Design review of the part built by this model. Coordinates are the model's own, in mm. Face numbers are marked on the shaded views. A direction names the side the tool comes from. Give positions to 0.01 mm unless a question says otherwise; leave off trailing zeros. Loops run counter-clockwise (first coordinate to the right, second up) from the corner with the lowest first, then second, coordinate; pieces in that order, holes last. Notation, with made-up numbers: (87, 21) - (143, 21) arc R24 ccw to (143, 39) - close; hole circle Ø7 at (55, 60.5). An arc over 180 degrees is marked (long way). Write each question's results on one line, items separated by ' | '.
```python
from build123d import *

# Parameters (mm, degrees)
SKETCH2_R           = 40
BOSS_EXTRUDE1_DEPTH = 20
SKETCH3_W           = 5.5
SKETCH3_H           = 4.31
SKETCH3_W_2         = 4.31
SKETCH3_H_2         = 5.5
CUT_EXTRUDE1_DEPTH  = 20
SKETCH4_R           = 6
CUT_EXTRUDE2_DEPTH  = 20


with BuildPart() as part:
    # Sketch2 → Boss-Extrude1 (new body)
    with BuildSketch(Plane.XY):
        Circle(SKETCH2_R)
    extrude(amount=BOSS_EXTRUDE1_DEPTH)

    # Sketch3 → Cut-Extrude1 (cut)
    with BuildSketch(Plane.XY):
        Polygon((-6.648248649, -35.436785829), (-7.763758734, -39.59992614), (-13.076350778, -38.176421392), (-11.960840694, -34.013281081), align=None)
        with Locations((0, -38.105)):
            Rectangle(SKETCH3_W, SKETCH3_H)
        Polygon((-15.59343014, -32.508613266), (-17.74843014, -36.241182756), (-22.51156986, -33.491182756), (-20.35656986, -29.758613266), align=None)
        Polygon((-23.475945135, -27.365032432), (-26.523575362, -30.412662659), (-30.412662659, -26.523575362), (-27.365032432, -23.475945135), align=None)
        Polygon((-29.758613266, -20.35656986), (-33.491182756, -22.51156986), (-36.241182756, -17.74843014), (-32.508613266, -15.59343014), align=None)
        Polygon((-34.013281081, -11.960840694), (-38.176421392, -13.076350778), (-39.59992614, -7.763758734), (-35.436785829, -6.648248649), align=None)
        with Locations((-38.105, 0)):
            Rectangle(SKETCH3_W_2, SKETCH3_H_2)
        Polygon((-35.436785829, 6.648248649), (-39.59992614, 7.763758734), (-38.176421392, 13.076350778), (-34.013281081, 11.960840694), align=None)
        Polygon((-32.508613266, 15.59343014), (-36.241182756, 17.74843014), (-33.491182756, 22.51156986), (-29.758613266, 20.35656986), align=None)
        Polygon((-27.365032432, 23.475945135), (-30.412662659, 26.523575362), (-26.523575362, 30.412662659), (-23.475945135, 27.365032432), align=None)
        Polygon((-20.35656986, 29.758613266), (-22.51156986, 33.491182756), (-17.74843014, 36.241182756), (-15.59343014, 32.508613266), align=None)
        Polygon((-11.960840694, 34.013281081), (-13.076350778, 38.176421392), (-7.763758734, 39.59992614), (-6.648248649, 35.436785829), align=None)
        with Locations((0, 38.105)):
            Rectangle(SKETCH3_W, SKETCH3_H)
        Polygon((6.648248649, 35.436785829), (7.763758734, 39.59992614), (13.076350778, 38.176421392), (11.960840694, 34.013281081), align=None)
        Polygon((15.59343014, 32.508613266), (17.74843014, 36.241182756), (22.51156986, 33.491182756), (20.35656986, 29.758613266), align=None)
        Polygon((23.475945135, 27.365032432), (26.523575362, 30.412662659), (30.412662659, 26.523575362), (27.365032432, 23.475945135), align=None)
        Polygon((29.758613266, 20.35656986), (33.491182756, 22.51156986), (36.241182756, 17.74843014), (32.508613266, 15.59343014), align=None)
        Polygon((34.013281081, 11.960840694), (38.176421392, 13.076350778), (39.59992614, 7.763758734), (35.436785829, 6.648248649), align=None)
        with Locations((38.105, 0)):
            Rectangle(SKETCH3_W_2, SKETCH3_H_2)
        Polygon((35.436785829, -6.648248649), (39.59992614, -7.763758734), (38.176421392, -13.076350778), (34.013281081, -11.960840694), align=None)
        Polygon((32.508613266, -15.59343014), (36.241182756, -17.74843014), (33.491182756, -22.51156986), (29.758613266, -20.35656986), align=None)
        Polygon((27.365032432, -23.475945135), (30.412662659, -26.523575362), (26.523575362, -30.412662659), (23.475945135, -27.365032432), align=None)
        Polygon((20.35656986, -29.758613266), (22.51156986, -33.491182756), (17.74843014, -36.241182756), (15.59343014, -32.508613266), align=None)
        Polygon((11.960840694, -34.013281081), (13.076350778, -38.176421392), (7.763758734, -39.59992614), (6.648248649, -35.436785829), align=None)
    extrude(amount=CUT_EXTRUDE1_DEPTH, mode=Mode.SUBTRACT)

    # Sketch4 → Cut-Extrude2 (cut)
    with BuildSketch(Plane.XY):
        Circle(SKETCH4_R)
    extrude(amount=CUT_EXTRUDE2_DEPTH, mode=Mode.SUBTRACT)


solid = part.part
```
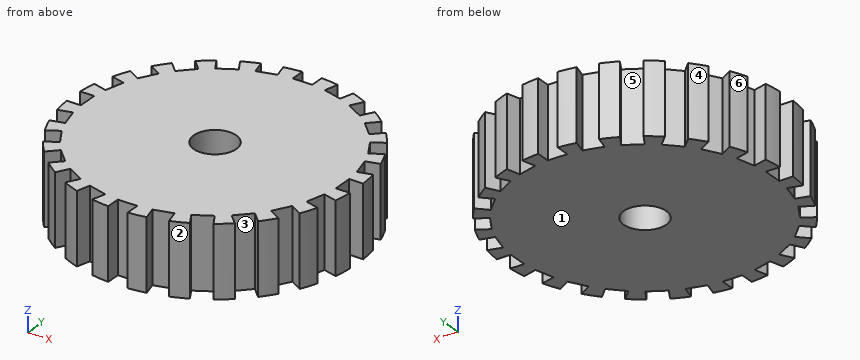
Item 1: Clearance check with flat-ended pins moving along their axes: P1, Ø2, axis at y = -22, z = 12.5, coming from the -X side; P2, Ø3, axis at y = 0.5, z = 9, coming from the +X side; P3, Ø4.5, axis at x = 0, z = 13, coming from the -Y side; P4, Ø12, axis at x = 28.5, y = -21, coming from the -Z side. State where each tip first meets the part, or that it passes through.
Output values:
P1: stops at x = -33.18 | P2: stops at x = 35.95 | P3: stops at y = -35.95 | P4: stops at z = 0
Item 2: We need section A-A on x = 0. Give the boundary of the cut face in (y, z).
Output values:
outline: (-35.95, 0) - (-6, 0) - (-6, 20) - (-35.95, 20) - close; (6, 0) - (35.95, 0) - (35.95, 20) - (6, 20) - close
Item 3: Wall thickness on probe 1 along Y at (x, z) = (24, 16); probe 2 along Y at (x, z) = (0, 11.5); probe 3 along Y at (x, z) = (-32.5, 17.5): over which ranges is each line inside the solid? List them lowest first.
Output values:
probe 1: y = -32 to -27.89, -26.84 to 26.84, 27.89 to 32 | probe 2: y = -35.95 to -6, 6 to 35.95 | probe 3: y = -23.32 to -21.94, -15.61 to 15.61, 21.94 to 23.32
Item 4: Draft analysis for pull direction Y (two halves, no side actions). For the marked faces 1, 2, 3 and 4, state which applies: +Y half, -Y half, draft (parallel to the pull), parting line (faces both ways), or undercut.
Output values:
face 1: draft | face 2: -Y half | face 3: undercut | face 4: +Y half
Item 5: Tool access review of the marked faces 5 and 6: name each direction out of +Z, -Z, +X, -X, +Y, -Y from which nothing blocks a thin tool from reaching the whole face with its end or side.
Output values:
face 5: +Z, -Z | face 6: +Z, -Z, -X, +Y
Item 6: We need section C-C on x = 14. Give the boundary of the cut face in (y, z), then the cut area to 3 significant figures.
Output values:
outline: (-37.47, 0) - (37.47, 0) - (37.47, 20) - (-37.47, 20) - close | area: 1,500 mm²
